Autodesk Inventor part; units mm, degrees
ref_plane "YZ Plane" through (0, 0, 0) normal (1, 0, 0) x (0, 1, 0)
ref_plane "XZ Plane" through (0, 0, 0) normal (0, 1, 0) x (-1, 0, 0)
ref_plane "XY Plane" through (0, 0, 0) normal (0, 0, 1) x (1, 0, 0)
sketch "Sketch1" plane through (0, 0, 0) normal (0, 0, 1) x (1, 0, 0)
  circle A0 centre (0, 0) radius 3.3
  circle A1 centre (-21.2, 0) radius 2
  line L0 (-21.2, 2) -> (0, 3.3)
  line L1 (0, -3.3) -> (-21.2, -2)
  dimension "d0" = 6.6
  dimension "d1" = 4
  dimension "d2" = 21.2
extrude "Extrusion1" add sketch "Sketch1" along normal blind 2 contours A0 L1 L0 | A0 L1 A1 L0 | A1
sketch "Sketch2" plane through (0, 0, 2) normal (0, 0, 1) x (1, 0, 0)
  arc A0 (0, -3.3) -> (0, 3.3) centre (0, 0) ccw
  circle A1 centre (0, 0) radius 3.3
  circle A2 centre (0, 0) radius 2.2
  dimension "d5" = 4.4
sketch "Sketch2 outline for Extrusion2" plane through (0, 0, 2) normal (0, 0, 1) x (1, 0, 0)
  arc A0 (0, 3.3) -> (0, -3.3) centre (0, 0) ccw
  arc A1 (0, -3.3) -> (0, 3.3) centre (0, 0) ccw
  circle A2 centre (0, 0) radius 2.2
extrude "Extrusion2" add sketch "Sketch2 outline for Extrusion2" along normal blind 2
sketch "Sketch3" plane through (0, 0, 4) normal (0, 0, 1) x (1, 0, 0)
  arc A0 (-0.403201, 3.275275) -> (-0.403201, -3.275275) centre (0, 0) ccw
  arc A1 (0, -3.3) -> (0, 3.3) centre (0, 0) ccw
  line L0 (-3.290517, 0.25) -> (3.290517, 0.25)
  line L1 (3.290517, 0.25) -> (3.290517, -0.25)
  line L2 (3.290517, -0.25) -> (-3.290517, -0.25)
  line L3 (-3.290517, -0.25) -> (-3.290517, 0.25)
  dimension "d8" = 0.25
  dimension "d9" = 0.25
extrude "Extrusion3" add sketch "Sketch3" along normal blind 1 contours L0 L1 L2 L3
properties part number "servo-swap"
Geometry check sheet. Reference: the model listing, model coordinates, mm. A direction names the side the tool comes from. Give positions to 0.01 mm unless a question says otherwise; leave off trailing zeros. Order: outer loops, then holes, each group sorted by start corner. A loop starts at its lowest first (then second) coordinate and runs counter-clockwise, first axis right, second up. Notation, with made-up numbers: (39.25, 59.25) - (68.25, 59.25) arc R22 cw to (68.25, 78.25) - close; hole circle Ø8 at (56.5, 47.5). An arc over 180 degrees is marked (long way). Write item = value, one per line. Start each with the question number.
1) Scan lines: L1, parallel to Y at x = 0, z = 3.5; L2, parallel to Z at x = -20.5, y = -0.25; L3, parallel to X at y = -1, z = 2.05. Record each from-to range of solid material in increasing order.
2) Draft check along X on faces 4 (the flat face through (0, 2.5, 4)), 5 (the flat face through (-10.45, -2.66, 0.99)), 6 (the flat face through (0, 0, 2)). Enter one of: released by +X, released by -X, zero draft, split by the parting line, or undercut.
3) Gauge pin test, flat ends, axial feed: pin 1 Ø1.5 at (y, z) = (-2, 2) entering from +X; pin 2 Ø0.8 at (x, z) = (1.5, 4.5) entering from +Y; pin 3 Ø1.1 at (x, z) = (-0.5, 4.5) entering from -Y. Record the tip position at first contact, or that the pin passes through.
4) Section check C-C (z = 2.55). Enter the section's corners in (x, y).
5) Section check B-B (x = 0.75). Enter the section's corners in (y, z), then the cut area to 3 significant figures.
6) Access from +Z, -Z, +X, -X, +Y, -Y to the whole of each face (thin tool, end or side, straight path). Record for faces 1 (the flat face through (0, 0.25, 4.5)), 2 (the flat face through (0, -2.4, 4)), 3 (the cylindrical face through (-23.2, 0, 1)).
7) Section check D-D (y = 1.5). Enter the section's corners in (x, z).
Geometry check:
q1.L1 = -3.3 to -2.2, 2.2 to 3.3
q1.L2 = 0 to 2
q1.L3 = -3.14 to -1.96, 1.96 to 3.14
q2.face_4 = zero draft
q2.face_5 = released by -X
q2.face_6 = undercut
q3.pin_1 = 3.05
q3.pin_2 = 0.25
q3.pin_3 = -3.29
q4.outline = circle Ø6.6 at (0, 0); hole circle Ø4.4 at (0, 0)
q5.outline = (-3.21, 0) - (3.21, 0) - (3.21, 4) - (2.07, 4) - (2.07, 2) - (-2.07, 2) - (-2.07, 4) - (-3.21, 4) - close; (-0.25, 4) - (0.25, 4) - (0.25, 5) - (-0.25, 5) - close
q5.area = 17.9 mm2
q6.face_1 = +Z, +X, -X, +Y
q6.face_2 = +Z, +X, -X, -Y
q6.face_3 = +Z, -Z, -X
q7.outline = (-22.52, 0) - (2.94, 0) - (2.94, 4) - (1.61, 4) - (1.61, 2) - (-1.61, 2) - (-1.61, 4) - (-2.94, 4) - (-2.94, 2) - (-22.52, 2) - close
